```python
from build123d import *

# Parameters (mm, degrees)
EXTRUDE_1_DEPTH   = 2
HOLE_WIZARD_M81_D = 9
CHAMFER_1_SIZE    = 2


with BuildPart() as part:
    # Эскиз1 → Бобышка-Вытянуть1 (new body)
    with BuildSketch(Plane(origin=(0, 0, 0), x_dir=(1, 0, 0), z_dir=(0, 0, -1))):
        Polygon((0, 0), (0, 135), (90, 135), (90, 90), (45, 90), (45, 0), align=None)
    extrude(amount=EXTRUDE_1_DEPTH)

    # Отверстие с зазором M81 (through all)
    with Locations(Plane(origin=(0, 0, -2), x_dir=(1, 0, 0), z_dir=(0, 0, -1))):
        with Locations((67.5, 112.5), (22.5, 112.5), (22.5, 67.5), (22.5, 22.5)):
            Hole(HOLE_WIZARD_M81_D / 2)

    # Фаска1
    chamfer_1_edges = [part.edges().sort_by_distance(p)[0] for p in [
        (0, 0, -1),
        (0, -135, -1),
        (90, -135, -1),
        (90, -90, -1),
        (45, 0, -1),
    ]]
    chamfer(chamfer_1_edges, length=CHAMFER_1_SIZE)


solid = part.part
```
Source: CAD feature listing. Evaluate the final solid. Frame: model axes, mm. Give positions to 0.01 mm unless a question says otherwise; leave off trailing zeros. Loops run counter-clockwise (first coordinate to the right, second up) from the corner with the lowest first, then second, coordinate; pieces in that order, holes last. Notation, with made-up numbers: (10.25, 8.25) -> (64.25, 8.25) arc R9 cw to (64.25, 21.25) -> close; hole circle Ø6 at (6.25, 31.5). An arc over 180 degrees is marked (long way). Use a Markdown table: item, result. Add a question column.
(1) Section query A-A (y = -67.5). Output: boundary loops of the cut face in (x, z), then the cut area to 3 significant figures.
(2) Pull-direction query (X, two-part tool) for faces 1 (the face through (25.82, -25.54, -0.99)), 2 (the face through (65.081, -116.294, -0.986)), 3 (the face through (36, -83, -2)); classes: +X half, -X half, draft (parallel to the pull), parting line (faces both ways), or undercut.
(3) Section query B-B (x = 22.5). Output: boundary loops of the cut face in (y, z).
(4) First-contact query: pin 1 Ø7 at (x, y) = (22.5, -22.5) entering from +Z; pin 2 Ø1 at (y, z) = (-53.5, -1) entering from +X. Flat tips, straight axial feed; report the tip coordinate or a pass-through.
(5) Section query C-C (y = -112.5). Output: boundary loops of the cut face in (x, z).
(6) Section query D-D (z = -0.6). Output: boundary loops of the cut face in (x, y).
(7) Ray query, line 1 (Y direction, x = 22.5, z = -1.4); line 2 (X direction, y = -112.5, z = -0.95); line 3 (X direction, y = -22.5, z = -1). Return the intervals inside material, ascending.
Checked values:
| question | item | result |
|---|---|---|
| 1 | outline | (0, -2) -> (18, -2) -> (18, 0) -> (0, 0) -> close; (27, -2) -> (45, -2) -> (45, 0) -> (27, 0) -> close |
| 1 | area | 72.0 mm^2 |
| 2 | face 1 | undercut |
| 2 | face 2 | undercut |
| 2 | face 3 | draft |
| 3 | outline | (-135, -2) -> (-117, -2) -> (-117, 0) -> (-135, 0) -> close; (-108, -2) -> (-72, -2) -> (-72, 0) -> (-108, 0) -> close; (-63, -2) -> (-27, -2) -> (-27, 0) -> (-63, 0) -> close; (-18, -2) -> (0, -2) -> (0, 0) -> (-18, 0) -> close |
| 4 | pin 1 | through |
| 4 | pin 2 | x = 45 |
| 5 | outline | (0, -2) -> (18, -2) -> (18, 0) -> (0, 0) -> close; (27, -2) -> (63, -2) -> (63, 0) -> (27, 0) -> close; (72, -2) -> (90, -2) -> (90, 0) -> (72, 0) -> close |
| 6 | outline | (0, -133) -> (2, -135) -> (88, -135) -> (90, -133) -> (90, -92) -> (88, -90) -> (45, -90) -> (45, -2) -> (43, 0) -> (2, 0) -> (0, -2) -> close; hole circle Ø9 at (22.5, -112.5); hole circle Ø9 at (22.5, -67.5); hole circle Ø9 at (22.5, -22.5); hole circle Ø9 at (67.5, -112.5) |
| 7 | line 1 | -135 to -117, -108 to -72, -63 to -27, -18 to 0 |
| 7 | line 2 | 0 to 18, 27 to 63, 72 to 90 |
| 7 | line 3 | 0 to 18, 27 to 45 |
